Autodesk Inventor part; units mm, degrees
ref_plane "YZ Plane" through (0, 0, 0) normal (1, 0, 0) x (0, 1, 0)
ref_plane "XZ Plane" through (0, 0, 0) normal (0, 1, 0) x (-1, 0, 0)
ref_plane "XY Plane" through (0, 0, 0) normal (0, 0, 1) x (1, 0, 0)
sketch "草图1" plane through (0, 0, 0) normal (0, 1, 0) x (-1, 0, 0)
  line L0 (0, 0) -> (65, 0)
  line L1 (65, 0) -> (65, -65)
  line L2 (65, -65) -> (0, -65)
  line L3 (0, -65) -> (0, 0)
  dimension "d0" = 65
  dimension "d1" = 65
extrude "拉伸1" add sketch "草图1" along normal blind 10
chamfer "倒角1" distance 65 angle 7 1 edges at (-32.5, 10, 0) measured on face at (-43.3333, 10, -43.3333)
sketch "草图2" plane through (0, 0, 0) normal (0, -1, 0) x (1, 0, 0)
  line L0 (-65, 0) -> (0, 0)
  line L1 (-32.5, 0) -> (-32.5, -65)
  line L2 (0, -65) -> (-65, -65)
  circle A0 centre (-32.5, -32.5) radius 1.95
  dimension "d7" = 3.9
extrude "拉伸2" cut sketch "草图2" against normal blind 4
sketch "草图3" plane through (0, 0, 0) normal (0, -1, 0) x (1, 0, 0)
  line L0 (0, -65) -> (-65, -65)
  line L1 (-65, -65) -> (-65, 0)
  line L2 (0, -65) -> (-65, -65)
  line L3 (-65, -65) -> (-65, -59)
  line L4 (-65, -59) -> (0, -59)
  line L5 (0, -59) -> (0, -65)
  point P0 (0, 0)
  dimension "d10" = 6
extrude "拉伸3" add sketch "草图3" along normal blind 50
sketch "草图4" plane through (-65, 10, -65) normal (0, 0.9925, 0.1219) x (1, 0, 0)
  line L0 (65, -7.3122) -> (65, 0)
  line L1 (65, 0) -> (62, 0)
  line L2 (62, 0) -> (62, -65.7342)
  line L3 (62, -65.7342) -> (65, -65.7342)
  line L4 (65, -65.7342) -> (65, 0)
  point P0 (65, -65.7342)
  dimension "d13" = 3
extrude "拉伸4" add sketch "草图4" along normal blind 65
sketch "草图5" plane through (0, 0, 0) normal (0, -1, 0) x (1, 0, 0)
  line L0 (-65, -59) -> (-65, -65)
  line L1 (0, 0) -> (-65, 0)
  line L2 (-65, 0) -> (-65, -59)
  line L3 (-65, -59) -> (0, -59)
  line L4 (0, -59) -> (0, 0)
extrude "拉伸5" add sketch "草图5" along normal blind 10
sketch "草图6" plane through (0, -10, 0) normal (0, -1, 0) x (1, 0, 0)
  circle A0 centre (-32.5, -32.5) radius 1.95
  circle A1 centre (-32.5, -32.5) radius 2.5
  point P0 (0, 0)
  dimension "d18" = 5
extrude "拉伸6" cut sketch "草图6" against normal blind 13 contours A0 | A1
equation "\"折弯半径\" = 厚度"
equation "\"折弯释压宽度\" = 厚度"
equation "\"折弯释压深度\" = 0.5 * 厚度"
equation "\"拐角释压尺寸\" = 4 * 厚度"
equation "\"最小余量\" = 2 * 厚度"
equation "\"过渡半径\" = 折弯半径"
equation "\"Jacobi半径尺寸\" = 折弯半径"
equation "\"间隙大小\" = 厚度"
properties part number "斜面"
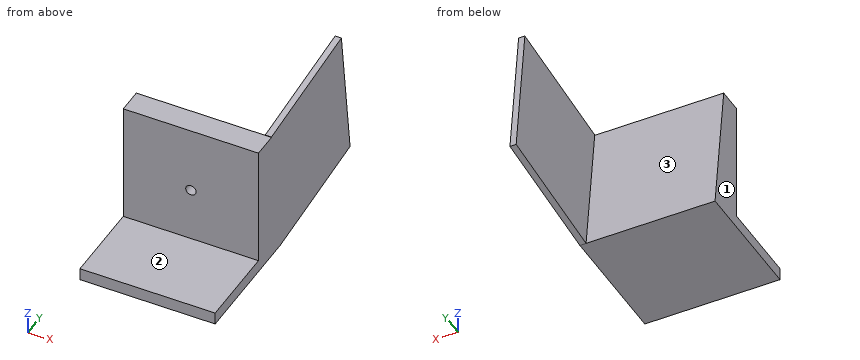
Input: part model. Units: mm. Frame: model coordinates. Face numbers are marked on the shaded views. A direction names the side the tool comes from. Coordinates: 2 decimals unless noted, no trailing zeros. Order: outer loops, then holes, each group sorted by start corner. A loop starts at its lowest first (then second) coordinate and runs counter-clockwise, first axis right, second up. Notation, with made-up numbers: (-16.5, 30) - (13.5, 30) arc R27 cw to (13.5, 54) - close; hole circle Ø6 at (-17, 69.25). An arc over 180 degrees is marked (long way). Return JSON: item names as keys, results as strings.
Q1. First-contact query: pin 1 (5.5 mm diameter, centred on x = -32, z = -33.5, fed in from -Y); pin 2 (22 mm diameter, centred on y = 55.5, z = -44, fed in from -X); pin 3 (4.5 mm diameter, centred on x = -32.5, z = -32.5, fed in from +Y). Flat tips, straight axial feed; report the tip coordinate or a pass-through.
The answers:
{"pin 1": "stops at y = -10", "pin 2": "stops at x = -3", "pin 3": "stops at y = 6.29"}
Q2. Cut plane A-A (y = -8). Return loops of the section in (x, z), then the cut area to 3 significant figures.
The answers:
{"outline": "(-65, -65) - (0, -65) - (0, 0) - (-65, 0) - close; hole circle Ø5 at (-32.5, -32.5)", "area": "4,210 mm2"}
Q3. Ray query, probe 1 along Z at (x, y) = (-5.5, -10.5); probe 2 along Y at (x, z) = (-50.5, -16); probe 3 along X at (y, z) = (23.5, -43). Return the intervals inside material, ascending.
The answers:
{"probe 1": "z = -65 to -59", "probe 2": "y = -10 to 3.98", "probe 3": "x = -3 to 0"}
Q4. Access query for the marked faces 1, 2 and 3. Directions: +Z, -Z, +X, -X, +Y, -Y. A direction counts if a zero-diameter tool reaches every point of the face in a straight line with its end or side. Return the directions, or none.
The answers:
{"face 1": "+Z, -Z, -X, +Y, -Y", "face 2": "+Z, +X, -X, -Y", "face 3": "+Z, -X, +Y"}
Q5. Cut plane C-C (z = -40). Return loops of the section in (x, y), then the cut area to 3 significant figures.
The answers:
{"outline": "(-65, -10) - (0, -10) - (0, 72.42) - (-3, 72.42) - (-3, 6.93) - (-65, 6.93) - close", "area": "1,300 mm2"}
